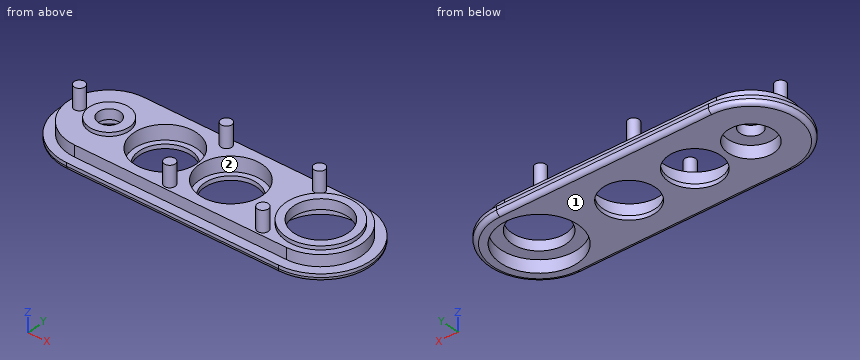
```python
from build123d import *

# Parameters (mm, degrees)
EXTRUDE_1_DEPTH     = 4.5
CUT_EXTRUDE_1_DEPTH = 2.7
SKETCH_3_R          = 2.6
SKETCH_3_R_2        = 6.5
SKETCH_3_R_3        = 6.25
CUT_EXTRUDE_2_DEPTH = 67.635200908
SKETCH_4_R          = 5.5
SKETCH_4_R_2        = 9.25
CUT_EXTRUDE_3_DEPTH = 3
FILLET_1_R          = 1
SKETCH_7_R          = 7.5
CUT_EXTRUDE_6_DEPTH = 3.5
SKETCH_9_R          = 1.3
EXTRUDE_2_DEPTH     = 5
EXTRUDE_START       = 0.9
SKETCH_10_R         = 4.8
SKETCH_10_R_2       = 2.6
SKETCH_10_R_3       = 8.3
SKETCH_10_R_4       = 6.5
EXTRUDE_3_DEPTH     = 0.9


with BuildPart() as part:
    # Эскиз1 → Бобышка-Вытянуть1 (new body)
    with BuildSketch(Plane.XY):
        with BuildLine():
            Line((0, 0), (50, 0))
            ThreePointArc((50, 0), (62, -12), (50, -24))
            Line((50, -24), (0, -24))
            ThreePointArc((0, -24), (-12, -12), (0, 0))
        make_face()
    extrude(amount=EXTRUDE_1_DEPTH)

    # Эскиз2 → Вырез-Вытянуть1 (cut)
    with BuildSketch(Plane.XY.offset(4.5)):
        with BuildLine():
            Line((0, 0.012347922), (50, 0.012347922))
            ThreePointArc((50, 0.012347922), (62.012347922, -12), (50, -24.012347922))
            Line((50, -24.012347922), (0, -24.012347922))
            ThreePointArc((0, -24.012347922), (-12.012347922, -12), (0, 0.012347922))
        make_face()
        with BuildLine():
            Line((0, -2.25), (50, -2.25))
            ThreePointArc((50, -2.25), (59.75, -12), (50, -21.75))
            Line((50, -21.75), (0, -21.75))
            ThreePointArc((0, -21.75), (-9.75, -12), (0, -2.25))
        make_face(mode=Mode.SUBTRACT)
    extrude(amount=-CUT_EXTRUDE_1_DEPTH, mode=Mode.SUBTRACT)

    # Эскиз3 → Вырез-Вытянуть2 (cut, through all)
    with BuildSketch(Plane.XY.offset(4.5)):
        with Locations((0, -12)):
            Circle(SKETCH_3_R)
        with Locations((50, -12)):
            Circle(SKETCH_3_R_2)
        with Locations((13.25, -12)):
            Circle(SKETCH_3_R_3)
        with Locations((28.75, -12)):
            Circle(SKETCH_3_R_3)
    extrude(amount=-CUT_EXTRUDE_2_DEPTH, mode=Mode.SUBTRACT)

    # Эскиз4 → Вырез-Вытянуть3 (cut)
    with BuildSketch(Plane(origin=(0, 0, 0), x_dir=(-1, 0, 0), z_dir=(0, 0, -1))):
        with Locations((0, -12)):
            Circle(SKETCH_4_R)
        with Locations((-50, -12)):
            Circle(SKETCH_4_R_2)
    extrude(amount=-CUT_EXTRUDE_3_DEPTH, mode=Mode.SUBTRACT)

    # Скругление1
    fillet_1_edges = [part.edges().sort_by_distance(p)[0] for p in [
        (25, 0, 0),
        (62, -12, 0),
        (25, -24, 0),
        (-12, -12, 0),
    ]]
    fillet(fillet_1_edges, radius=FILLET_1_R)

    # Эскиз7 → Вырез-Вытянуть6 (cut)
    with BuildSketch(Plane.XY.offset(4.5)):
        with Locations((28.75, -12)):
            Circle(SKETCH_7_R)
        with Locations((13.25, -12)):
            Circle(SKETCH_7_R)
    extrude(amount=-CUT_EXTRUDE_6_DEPTH, mode=Mode.SUBTRACT)

    # Эскиз9 → Бобышка-Вытянуть2 (add)
    with BuildSketch(Plane.XY.offset(4.5)):
        with Locations((21, -4)):
            Circle(SKETCH_9_R)
        with Locations((21, -20)):
            Circle(SKETCH_9_R)
        with Locations((-7, -12)):
            Circle(SKETCH_9_R)
        with Locations((43, -4)):
            Circle(SKETCH_9_R)
        with Locations((43, -20)):
            Circle(SKETCH_9_R)
    extrude(amount=EXTRUDE_2_DEPTH)

    # Эскиз10 → Бобышка-Вытянуть3 (add)
    # profile 1 of 2: a face of its own
    with BuildSketch(Plane.XY.offset(4.5).offset(EXTRUDE_START)):
        with Locations((0, -12)):
            Circle(SKETCH_10_R)
        with Locations((0, -12)):
            Circle(SKETCH_10_R_2, mode=Mode.SUBTRACT)
    # profile 2 of 2: a face of its own
    with BuildSketch(Plane.XY.offset(4.5).offset(EXTRUDE_START)):
        with Locations((50, -12)):
            Circle(SKETCH_10_R_3)
        with Locations((50, -12)):
            Circle(SKETCH_10_R_4, mode=Mode.SUBTRACT)
    extrude(amount=-EXTRUDE_3_DEPTH)


solid = part.part
```
Geometry check sheet. Reference: the model listing, model coordinates, mm. Face numbers are marked on the shaded views. Round coordinates to 2 decimals unless told otherwise and drop trailing zeros. Order: outer loops, then holes, each group sorted by start corner. A loop starts at its lowest first (then second) coordinate and runs counter-clockwise, first axis right, second up. Notation, with made-up numbers: (-23, -6) - (30, -6) arc R21 ccw to (30, 1) - close; hole circle Ø10 at (35, 57.25). An arc over 180 degrees is marked (long way). Use a Markdown table: item, result. Add a question column.
(1) Release check for a two-part mould opening along Y. For the marked faces 1 and 2 record: pulls with the +Y half, pulls with the -Y half, needs draft (parallel to the pull), parting line crosses it, or undercut.
(2) Depth check by flat-ended pin: pin 1 (1.4 mm diameter, centred on x = 24.5, z = 3, fed in from -Y); pin 2 (7 mm diameter, centred on x = 30, y = -14.5, fed in from +Z); pin 3 (3 mm diameter, centred on x = 2, y = -12.5, fed in from +Z); pin 4 (9 mm diameter, centred on x = 54, y = -15, fed in from -Z). Enter the tip coordinate at first touch or a pass-through.
(3) Material ranges on line 1 along X through (y, z) = (-12.5, 4); line 2 along Y through (x, z) = (13.25, 1.7); line 3 along X through (y, z) = (-11, 2.5), recorded low to high. Write a range as [from, to].
(4) Sectioned sample at A-A, the plane x = 28.75. Enter the section's corners in (y, z), and give its area (3 significant figures).
(5) Sectioned sample at B-B, the plane y = -12. Count the separate pieces of the cut face and the enclosed holes in it, and give its area (3 significant figures).
Answers below:
| question | item | result |
|---|---|---|
| 1 | face 1 | needs draft |
| 1 | face 2 | undercut |
| 2 | pin 1 | y = -21.75 |
| 2 | pin 2 | z = 1 |
| 2 | pin 3 | z = 5.4 |
| 2 | pin 4 | z = 0 |
| 3 | line 1 | [-9.74, -2.55], [2.55, 5.77], [20.73, 21.27], [36.23, 43.52], [56.48, 59.74] |
| 3 | line 2 | [-24, -19.5], [-4.5, 0] |
| 3 | line 3 | [-9.7, -5.41], [5.41, 5.82], [20.68, 21.32], [36.18, 40.8], [59.2, 59.7] |
| 4 | outline | (-24, 1) arc R1 ccw to (-23, 0) - (-18.25, 0) - (-18.25, 1) - (-19.5, 1) - (-19.5, 4.5) - (-21.75, 4.5) - (-21.75, 1.8) - (-24, 1.8) - close; (-5.75, 0) - (-1, 0) arc R1 ccw to (0, 1) - (0, 1.8) - (-2.25, 1.8) - (-2.25, 4.5) - (-4.5, 4.5) - (-4.5, 1) - (-5.75, 1) - close |
| 4 | area | 30.4 mm² |
| 5 | separate pieces | 5 |
| 5 | enclosed holes | 0 |
| 5 | area | 94.8 mm² |
